```python
from build123d import *

# Parameters (mm, degrees)
CROQUIS2_R                 = 1.5
CROQUIS2_R_2               = 6
SALIENTE_EXTRUIR2_DEPTH    = 2.7
CROQUIS3_R                 = 1.5
CROQUIS3_W                 = 2
CROQUIS3_H                 = 4
CORTAR_EXTRUIR1_DEPTH      = 1.0000001
CORTAR_EXTRUIR1_DEPTH_BACK = 3.7000001


with BuildPart() as part:
    # Croquis2 → Saliente-Extruir2 (new body)
    with BuildSketch(Plane.XY):
        with BuildLine():
            Line((-10.5, 28.115792599), (-10.5, 37.559952077))
            ThreePointArc((-10.5, 37.559952077), (-19.5, 33.774990748), (-27.277872663, 27.873242778))
            Line((-27.277872663, 27.873242778), (-19.098990638, 23.151163039))
            add(Edge.make_bspline(
                [(-29.598990638, 4.96462956), (-22.416381166, 12.9421037), (-19.098990638, 23.151163039)],
                knots=[0, 0, 0, 1, 1, 1], degree=2))
            Line((-29.598990638, 4.96462956), (-37.777872663, 9.686709299))
            ThreePointArc((-37.777872663, 9.686709299), (-39, 0), (-37.777872663, -9.686709299))
            Line((-37.777872663, -9.686709299), (-29.598990638, -4.96462956))
            add(Edge.make_bspline(
                [(-19.098990638, -23.151163039), (-22.416381166, -12.9421037), (-29.598990638, -4.96462956)],
                knots=[0, 0, 0, 1, 1, 1], degree=2))
            Line((-19.098990638, -23.151163039), (-27.277872663, -27.873242778))
            ThreePointArc((-27.277872663, -27.873242778), (-19.5, -33.774990748), (-10.5, -37.559952077))
            Line((-10.5, -37.559952077), (-10.5, -28.115792599))
            add(Edge.make_bspline(
                [(10.5, -28.115792599), (0, -25.884207401), (-10.5, -28.115792599)],
                knots=[0, 0, 0, 1, 1, 1], degree=2))
            Line((10.5, -28.115792599), (10.5, -37.559952077))
            ThreePointArc((10.5, -37.559952077), (19.5, -33.774990748), (27.277872663, -27.873242778))
            Line((27.277872663, -27.873242778), (19.098990638, -23.151163039))
            add(Edge.make_bspline(
                [(29.598990638, -4.96462956), (22.416381166, -12.9421037), (19.098990638, -23.151163039)],
                knots=[0, 0, 0, 1, 1, 1], degree=2))
            Line((29.598990638, -4.96462956), (37.777872663, -9.686709299))
            ThreePointArc((37.777872663, -9.686709299), (38.693261906, -4.88175), (39, 0))
            ThreePointArc((39, 0), (38.693261906, 4.88175), (37.777872663, 9.686709299))
            Line((37.777872663, 9.686709299), (29.598990638, 4.96462956))
            add(Edge.make_bspline(
                [(19.098990638, 23.151163039), (22.416381166, 12.9421037), (29.598990638, 4.96462956)],
                knots=[0, 0, 0, 1, 1, 1], degree=2))
            Line((19.098990638, 23.151163039), (27.277872663, 27.873242778))
            ThreePointArc((27.277872663, 27.873242778), (19.5, 33.774990748), (10.5, 37.559952077))
            Line((10.5, 37.559952077), (10.5, 28.115792599))
            add(Edge.make_bspline(
                [(-10.5, 28.115792599), (0, 25.884207401), (10.5, 28.115792599)],
                knots=[0, 0, 0, 1, 1, 1], degree=2))
        make_face()
        with Locations((-17.142037335, -29.69087961)):
            Circle(CROQUIS2_R, mode=Mode.SUBTRACT)
        with Locations((-34.28407467, 0)):
            Circle(CROQUIS2_R, mode=Mode.SUBTRACT)
        with Locations((17.142037335, -29.69087961)):
            Circle(CROQUIS2_R, mode=Mode.SUBTRACT)
        with Locations((-17.142037335, 29.69087961)):
            Circle(CROQUIS2_R, mode=Mode.SUBTRACT)
        Circle(CROQUIS2_R_2, mode=Mode.SUBTRACT)
        with Locations((34.28407467, 0)):
            Circle(CROQUIS2_R, mode=Mode.SUBTRACT)
        with Locations((17.142037335, 29.69087961)):
            Circle(CROQUIS2_R, mode=Mode.SUBTRACT)
    extrude(amount=SALIENTE_EXTRUIR2_DEPTH)

    # Croquis3 → Cortar-Extruir1 (cut, two sides)
    with BuildSketch(Plane.XY.offset(2.7)) as cortar_extruir1_sk:
        with Locations((9.526279442, 5.5)):
            Circle(CROQUIS3_R)
        with Locations((5.5, -9.526279442)):
            Circle(CROQUIS3_R)
        with Locations((-9.526279442, -5.5)):
            Circle(CROQUIS3_R)
        with Locations((-5.5, 9.526279442)):
            Circle(CROQUIS3_R)
        with Locations((-11.5, 34.5)):
            Rectangle(CROQUIS3_W, CROQUIS3_H)
        with Locations((11.5, 34.5)):
            Rectangle(CROQUIS3_W, CROQUIS3_H)
        Polygon((22.895825623, 25.34326674), (21.895825623, 27.075317547), (25.359927238, 29.075317547), (26.359927238, 27.34326674), align=None)
        Polygon((36.859927238, 9.15673326), (37.859927238, 7.424682453), (34.395825623, 5.424682453), (33.395825623, 7.15673326), align=None)
        Polygon((33.395825623, -7.15673326), (34.395825623, -5.424682453), (37.859927238, -7.424682453), (36.859927238, -9.15673326), align=None)
        Polygon((26.359927238, -27.34326674), (25.359927238, -29.075317547), (21.895825623, -27.075317547), (22.895825623, -25.34326674), align=None)
        with Locations((11.5, -34.5)):
            Rectangle(CROQUIS3_W, CROQUIS3_H)
        with Locations((-11.5, -34.5)):
            Rectangle(CROQUIS3_W, CROQUIS3_H)
        Polygon((-22.895825623, -25.34326674), (-21.895825623, -27.075317547), (-25.359927238, -29.075317547), (-26.359927238, -27.34326674), align=None)
        Polygon((-36.859927238, -9.15673326), (-37.859927238, -7.424682453), (-34.395825623, -5.424682453), (-33.395825623, -7.15673326), align=None)
        Polygon((-33.395825623, 7.15673326), (-34.395825623, 5.424682453), (-37.859927238, 7.424682453), (-36.859927238, 9.15673326), align=None)
        Polygon((-26.359927238, 27.34326674), (-25.359927238, 29.075317547), (-21.895825623, 27.075317547), (-22.895825623, 25.34326674), align=None)
    extrude(amount=CORTAR_EXTRUIR1_DEPTH, mode=Mode.SUBTRACT)
    extrude(cortar_extruir1_sk.sketch, amount=-CORTAR_EXTRUIR1_DEPTH_BACK, mode=Mode.SUBTRACT)


solid = part.part
```
Geometry check sheet. Reference: the model listing, model coordinates, mm. A direction names the side the tool comes from. Coordinates: 2 decimals unless noted, no trailing zeros.
Item 1: Release check for a two-part mould opening along Y. For faces 1 (the face through (-31.471, 6.045, 1.331)), 2 (the face through (-12.5, -35, 1)), 3 (the face through (8, 1, 0)) record: released by +Y, released by -Y, zero draft, split by the parting line, or undercut.
Item 2: Sectioned sample at A-A, the plane z = 1.05. Count the separate pieces of the cut face and the enclosed holes in it, then the cut area to 3 significant figures.
Item 3: Access from +Z, -Z, +X, -X, +Y, -Y to the whole of each face (thin tool, end or side, straight path). Record for faces 4 (the face through (-22.4, -26.2, 1.4)), 5 (the face through (36.152, 6.439, 1.369)), 6 (the face through (10.5, -30, 1)).
Item 4: Thickness scan on line 1 (Y direction, x = 5, z = 2.5); line 2 (X direction, y = -29.5, z = 2.35); line 3 (Y direction, x = 25, z = 2.35). Record the ranges inside material, lowest first.
Item 5: Go/stop test with flat-tipped pins: pin 1 Ø2.5 at (x, y) = (9.53, 5.5) entering from -Z; pin 2 Ø0.8 at (y, z) = (-35.5, 2) entering from +X; pin 3 Ø1.6 at (x, z) = (-11.5, 1) entering from +Y; pin 4 Ø1.5 at (x, z) = (15.5, 1) entering from +Y. Record where each tip stops, or that it passes through.
Check result:
1. face 1: released by +Y
1. face 2: undercut
1. face 3: zero draft
2. separate pieces: 1
2. enclosed holes: 11
2. area: 3,090 mm2
3. face 4: +Z, -Z, -X
3. face 5: +Z, -Z
3. face 6: +Z, -Z, -Y
4. line 1: y = -27.25 to -10.94, -8.11 to -3.32, 3.32 to 27.25
4. line 2: x = -25.51 to -18.63, -15.65 to -10.5, 10.5 to 15.65, 18.63 to 25.51
4. line 3: y = -29.93 to -28.87, -10.89 to 10.89, 28.87 to 29.93
5. pin 1: passes through
5. pin 2: stops at x = 17
5. pin 3: stops at y = 37.5
5. pin 4: stops at y = 36.1
